Work out the finished part from the listing and answer in its coordinate system (mm). A direction names the side the tool comes from. Coordinates: 2 decimals unless noted, no trailing zeros. Order: outer loops, then holes, each group sorted by start corner. A loop starts at its lowest first (then second) coordinate and runs counter-clockwise, first axis right, second up. Notation, with made-up numbers: (-30.5, 30.25) -> (23.5, 30.25) arc R16 cw to (23.5, 39.25) -> close; hole circle Ø2 at (74.25, 28.5). An arc over 180 degrees is marked (long way). Answer as CSV lines item,"result". Start each with the question number.
Item 1: Which of the six approach directions +Z, -Z, +X, -X, +Y, -Y give full straight-line access (tool end or side, diameter ignored) to faces 1 (the face through (23, 40, 50)), 2 (the face through (49, 30, 0)), 3 (the face through (41.301, 49.312, 20.998))?
Item 2: For a pull along Y with two mould halves and no side action, classify faces 4 (the face through (77, 30, 23)), 5 (the face through (49, 0, 10)), 6 (the face through (36.66, 48.75, 30.12)) as pulls with the +Y half, pulls with the -Y half, needs draft (parallel to the pull), parting line crosses it, or undercut.
Item 3: Section B-B (z = 23) is taken. Write down the section's boundary in (x, y).
Item 4: Each of these flat-tipped pins is pushed along its axis until it touches: pin 1 Ø1.5 at (x, z) = (20, 51) entering from -Y; pin 2 Ø16 at (x, y) = (42.5, 7) entering from +Z; pin 3 Ø6 at (x, y) = (37.5, 26.5) entering from +Z. Where does it stop, or does it pass through?
Item 5: Section A-A (x = 34) is taken. Write down the section's boundary in (y, z).
Item 6: Section D-D (y = 28.5) is taken. Write down the section's boundary in (x, z).
Item 7: Section C-C (y = 42) is taken. Write down the section's boundary in (x, z).
Item 8: Straight lines are drawn through the part: L1, parallel to Z at x = 60, y = 21; L2, parallel to Z at x = 19, y = 6.5; L3, parallel to Z at x = 55.5, y = 34.5. For each, find the intervals that lie inside material, in ascending order.
```python
from build123d import *

# Parameters (mm, degrees)
F1_DEPTH = 100
F3_DEPTH = 60.001
F5_DEPTH = 100.001


with BuildPart() as f1:
    # F0 (on Right) → F1 (new body)
    with BuildSketch(Plane.YZ):
        Polygon((0, 20), (0, 0), (60, 0), (60, 60), (40, 60), (40, 40), (20, 40), (20, 20), align=None)
    extrude(amount=F1_DEPTH)

    # F2 (on face) → F3 (cut, through all)
    with BuildSketch(Plane(origin=(0, 60, 0), x_dir=(-1, 0, 0), z_dir=(0, 1, 0))):
        Polygon((-100, 60), (-100, 0), (-40.003979, 60), align=None)
    extrude(amount=-F3_DEPTH, mode=Mode.SUBTRACT)

    # F4 (on face) → F5 (cut, through all)
    with BuildSketch(Plane(origin=(0, 0, 0), x_dir=(0, -1, 0), z_dir=(-1, 0, 0))):
        Polygon((-30.586883, 24.511646), (-35.370231, 33.922151), (-45.91164, 34.484902), (-51.669702, 25.63715), (-46.886355, 16.226646), (-36.344945, 15.663894), align=None)
    extrude(amount=-F5_DEPTH, mode=Mode.SUBTRACT)


solid = f1.part
```
Checked values:
1,face 1,"+Z, +X, -X, -Y"
1,face 2,"-Z, +X, -X, +Y, -Y"
1,face 3,"+X, -X"
2,face 4,"needs draft"
2,face 5,"pulls with the -Y half"
2,face 6,"undercut"
3,outline,"(0, 20) -> (77, 20) -> (77, 31.57) -> (0, 31.57) -> close; (0, 50.33) -> (77, 50.33) -> (77, 60) -> (0, 60) -> close"
4,pin 1,"stops at y = 40"
4,pin 2,"stops at z = 20"
4,pin 3,"stops at z = 40"
5,outline,"(0, 0) -> (60, 0) -> (60, 60) -> (40, 60) -> (40, 40) -> (20, 40) -> (20, 20) -> (0, 20) -> close; hole (30.59, 24.51) -> (36.34, 15.66) -> (46.89, 16.23) -> (51.67, 25.64) -> (45.91, 34.48) -> (35.37, 33.92) -> close"
6,outline,"(0, 0) -> (100, 0) -> (60, 40) -> (0, 40) -> close"
7,outline,"(0, 0) -> (100, 0) -> (84.04, 15.97) -> (0, 15.97) -> close; (0, 34.28) -> (65.73, 34.28) -> (40, 60) -> (0, 60) -> close"
8,L1,"z = 0 to 40"
8,L2,"z = 0 to 20"
8,L3,"z = 0 to 18.5, 32.21 to 40"
